Geometry: final body of the model. Coordinates: model frame, mm. Give positions to 0.01 mm unless a question says otherwise; leave off trailing zeros. Order: outer loops, then holes, each group sorted by start corner. A loop starts at its lowest first (then second) coordinate and runs counter-clockwise, first axis right, second up. Notation, with made-up numbers: (37, 39) -> (92, 39) arc R22 cw to (92, 63) -> close; hole circle Ø6 at (29.25, 87.25). An arc over 180 degrees is marked (long way). One line per item, written item: value. Start each with the question number.
```python
from build123d import *

# Parameters (mm, degrees)
F0_W     = 113.6151142418
F0_H     = 109.588842839
F1_DEPTH = 105.6814342737
F2_R     = 24.0827135545
F3_DEPTH = 200


# Not quite as in the source:
# - the program builds the solid bodies; features that only make, move or delete a surface that nothing else refers to are left out


with BuildPart() as f1:
    # F0 (on Top) → F1 (new body)
    with BuildSketch(Plane.XY):
        with Locations((-3.817750141, 19.6385178715)):
            Rectangle(F0_W, F0_H)
    extrude(amount=F1_DEPTH)

    # F2 (on face) → F3 (cut)
    with BuildSketch(Plane.YZ.offset(52.9898069799)):
        with Locations((38.0479171872, 52.4106435478)):
            Circle(F2_R)
    extrude(amount=-F3_DEPTH, mode=Mode.SUBTRACT)


solid = f1.part
```
1. Draft query along Z for faces 1 (the cylindrical face through (-3, 60.3, 43.2)), 2 (the flat face through (-5, 20, 0)), 3 (the flat face through (52.99, 7, 52)), 4 (the flat face through (-5, 20, 105.681)). Return one class per face: pulls with the +Z half, pulls with the -Z half, needs draft (parallel to the pull), parting line crosses it, or undercut.
2. Cut plane B-B, the plane y = 51. Return loops of the section in (x, z).
3. Cut plane A-A, the plane z = 34.5. Return loops of the section in (x, y), then the cut area to 3 significant figures.
4. Material intervals for L1, parallel to Y at x = 41, z = 51.5; L2, parallel to Z at x = -45, y = 53; L3, parallel to Z at x = -42, y = 22, sorted ascending. Write a range as [from, to].
5. Cut plane C-C, the plane x = 42. Return loops of the section in (y, z).
Answers follow:
1. face 1: undercut
1. face 2: pulls with the -Z half
1. face 3: needs draft
1. face 4: pulls with the +Z half
2. outline: (-60.63, 0) -> (52.99, 0) -> (52.99, 32.11) -> (-60.63, 32.11) -> close; (-60.63, 72.71) -> (52.99, 72.71) -> (52.99, 105.68) -> (-60.63, 105.68) -> close
3. outline: (-60.63, -35.16) -> (52.99, -35.16) -> (52.99, 21.95) -> (-60.63, 21.95) -> close; (-60.63, 54.15) -> (52.99, 54.15) -> (52.99, 74.43) -> (-60.63, 74.43) -> close
3. area: 8,790 mm²
4. L1: y = [-35.16, 13.98], [62.11, 74.43]
4. L2: z = [0, 33.53], [71.29, 105.68]
4. L3: z = [0, 34.45], [70.37, 105.68]
5. outline: (-35.16, 0) -> (74.43, 0) -> (74.43, 105.68) -> (-35.16, 105.68) -> close; hole circle Ø48.17 at (38.05, 52.41)
